Input: part model. Units: mm. Frame: model coordinates. A direction names the side the tool comes from. Coordinates: 2 decimals unless noted, no trailing zeros. Write each loop counter-clockwise with the first axis right and the second up, starting at its lowest first coordinate (ties: lowest second). Pieces come first, ordered by that corner, then holes. Notation, with made-up numbers: M -31.75,-8 L -2.75,-8 A17 cw -2.75,1 Z; hole C -1,-25 d6. An arc over 180 degrees is marked long. Use one line per item in the form item = value.
from build123d import *

# Parameters (mm, degrees)
F1_DEPTH = 2.159
F5_W     = 53.7838474663
F5_H     = 6.096
F5_W_2   = 50.7808425279


with BuildPart() as f1:
    # F0 (on Top) → F1 (new body)
    with BuildSketch(Plane.XY):
        with BuildLine():
            Line((-27.1301528547, -3.0107952586), (-27.1301528547, -6.8207952586))
            Line((-27.1301528547, -6.8207952586), (99.8698471453, -6.8207952586))
            Line((99.8698471453, -6.8207952586), (99.8698471453, 28.7392047414))
            Line((99.8698471453, 28.7392047414), (-27.1301528547, 28.7392047414))
            Line((-27.1301528547, 28.7392047414), (-27.1301528547, 24.9292047414))
            ThreePointArc((-27.1301528547, 24.9292047414), (-13.1601528547, 10.9592047414), (-27.1301528547, -3.0107952586))
        make_face()
    extrude(amount=F1_DEPTH)

    # F5 (on 3pt) → F6 (join, up to the next surface of F1)
    with BuildSketch(Plane(origin=(2.9275761968, 0, 17.9605901646), x_dir=(0.9869744889, 0, -0.1608768417), z_dir=(0.1608768417, 0, 0.9869744889))):
        with Locations((71.3297345118, -3.7727952586)):
            Rectangle(F5_W, F5_H)
        with Locations((72.8312369809, 25.6912047414)):
            Rectangle(F5_W_2, F5_H)
    extrude(until=Until.NEXT, dir=(-0.1608768417, 0, -0.9869744889))


solid = f1.part
(1) Section query C-C on y = 18. Return the cut outline in (x, z), plus the area to 3 significant figures.
Computed:
outline = M -15.06,0 L 99.87,0 L 99.87,2.16 L -15.06,2.16 Z
area = 248 mm^2
(2) Section query B-B on x = 55. Return the cut outline in (y, z).
Computed:
outline = M -6.82,0 L 28.74,0 L 28.74,9.47 L 22.64,9.47 L 22.64,2.16 L -0.72,2.16 L -0.72,9.47 L -6.82,9.47 Z
(3) Section query D-D on x = 73. Return the cut outline in (y, z).
Computed:
outline = M -6.82,0 L 28.74,0 L 28.74,6.54 L 22.64,6.54 L 22.64,2.16 L -0.72,2.16 L -0.72,6.54 L -6.82,6.54 Z
(4) Section query A-A on z = 6.75. Return the cut outline in (x, y), plus the area to 3 significant figures.
Computed:
outline = M 46.12,-6.82 L 71.7,-6.82 L 71.7,-0.72 L 46.12,-0.72 Z; M 49.17,22.64 L 71.7,22.64 L 71.7,28.74 L 49.17,28.74 Z
area = 293 mm^2
(5) Pull-direction query (Y, two-part tool) for faces 6 (the flat face through (99.87, 11, 1)), 7 (the flat face through (68, 22.643, 4)), 8 (the flat face through (51, 28.739, 3)); classes: pulls with the +Y half, pulls with the -Y half, needs draft (parallel to the pull), parting line crosses it, or undercut.
Computed:
face_6 = needs draft
face_7 = undercut
face_8 = pulls with the +Y half
(6) Set-up query: faces 1 (the flat face through (72.957, -3.73, 6.546)), 2 (the flat face through (-27.13, 27, 1)), 3 (the flat face through (49.094, 25.649, 6.301)), 4 (the flat face through (35, 11, 2.159)), 5 (the flat face through (67, -0.725, 4)). Return all of +Z, -Z, +X, -X, +Y, -Y with unobstructed straight access to the full face (end or side cutting, diameter ignored); none if empty.
Computed:
face_1 = +Z, +X, +Y, -Y
face_2 = +Z, -Z, -X, +Y, -Y
face_3 = +Z, -X, +Y
face_4 = +Z, -X
face_5 = +Z, +X, -X
(7) Line query: probe 1 along Y at (x, z) = (78.5, 4.5); probe 2 along Z at (x, y) = (-13.5, 19.5); probe 3 along X at (y, z) = (16, 0.75). Output: solid intervals per line, ascending.
Computed:
probe_1 = -6.82 to -0.72, 22.64 to 28.74
probe_2 = 0 to 2.16
probe_3 = -14.1 to 99.87
(8) First-contact query: pin 1 Ø18 at (x, y) = (45.5, 4.5) entering from +Z; pin 2 Ø3 at (y, z) = (24, 7.5) entering from -X; pin 3 Ø1 at (x, y) = (1, 21) entering from +Z. Flat tips, straight axial feed; report the tip coordinate or a pass-through.
Computed:
pin_1 = 10.81
pin_2 = 49.04
pin_3 = 2.16
